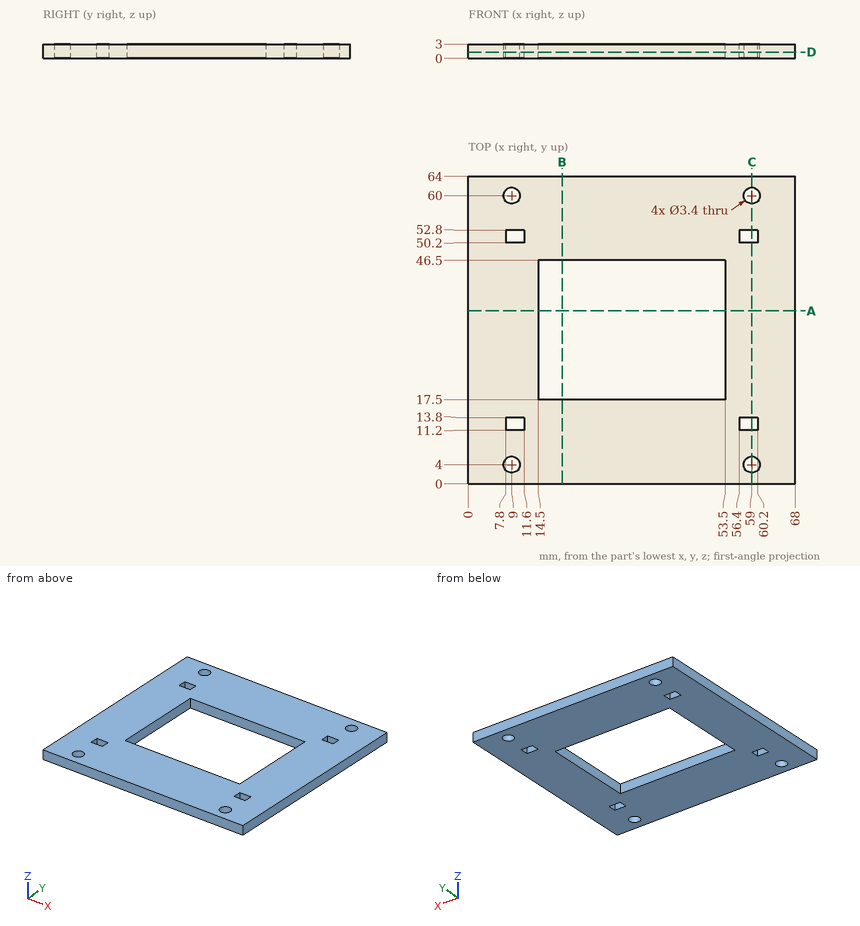
Can you work these out from the drawing? Everything is in mm from the part's minimum corner. Round coordinates to 2 decimals unless told otherwise and drop trailing zeros. Loops run counter-clockwise (first coordinate to the right, second up) from the corner with the lowest first, then second, coordinate; pieces in that order, holes last. Notation, with made-up numbers: (76, -24) -> (96, -24) arc R9 cw to (96, -19) -> close; hole circle Ø8 at (5.25, -7). An arc over 180 degrees is marked (long way). Use CSV: the item, a comma, the result in double quotes.
(1) Suppose I cut it at D-D on z = 1.3. Give the number of separate pieces and of enclosed holes in the cut face, plus the area to 3 significant figures.
Return value:
separate pieces,"1"
enclosed holes,"9"
area,"3,150 mm²"
(2) If I drill on probe 1 along Y at (x, z) = (59, 1.3); probe 2 along X at (y, z) = (4, 0.7); probe 3 along Y at (x, z) = (36, 0.2), over which ranges is the centre line in solid material (lowest first)? Write a range as [from, to].
Return value:
probe 1,"y = [0, 2.3], [5.7, 11.2], [13.8, 50.2], [52.8, 58.3], [61.7, 64]"
probe 2,"x = [0, 7.3], [10.7, 57.3], [60.7, 68]"
probe 3,"y = [0, 17.5], [46.5, 64]"
(3) Suppose I cut it at A-A on y = 36. Write out the boundary of the cut face in (x, z), plus the area to 3 significant figures.
Return value:
outline,"(0, 0) -> (14.5, 0) -> (14.5, 3) -> (0, 3) -> close; (53.5, 0) -> (68, 0) -> (68, 3) -> (53.5, 3) -> close"
area,"87.0 mm²"
(4) Suppose I cut it at B-B on x = 19.5. Write out the boundary of the cut face in (y, z).
Return value:
outline,"(0, 0) -> (17.5, 0) -> (17.5, 3) -> (0, 3) -> close; (46.5, 0) -> (64, 0) -> (64, 3) -> (46.5, 3) -> close"
(5) Will this pin go through, and if not, where does the flat tip stop? pin 1 Ø3 at (x, y) = (9, 4) entering from +Z.
Return value:
pin 1,"passes through"
(6) Suppose I cut it at C-C on x = 59. Write out the boundary of the cut face in (y, z).
Return value:
outline,"(0, 0) -> (2.3, 0) -> (2.3, 3) -> (0, 3) -> close; (5.7, 0) -> (11.2, 0) -> (11.2, 3) -> (5.7, 3) -> close; (13.8, 0) -> (50.2, 0) -> (50.2, 3) -> (13.8, 3) -> close; (52.8, 0) -> (58.3, 0) -> (58.3, 3) -> (52.8, 3) -> close; (61.7, 0) -> (64, 0) -> (64, 3) -> (61.7, 3) -> close"
